Could you check a few things on this drawing? It's one solid part, dimensions in mm from its lowest x, y, z. A direction names the side the tool comes from. Coordinates: 2 decimals unless noted, no trailing zeros. Order: outer loops, then holes, each group sorted by start corner. A loop starts at its lowest first (then second) coordinate and runs counter-clockwise, first axis right, second up.
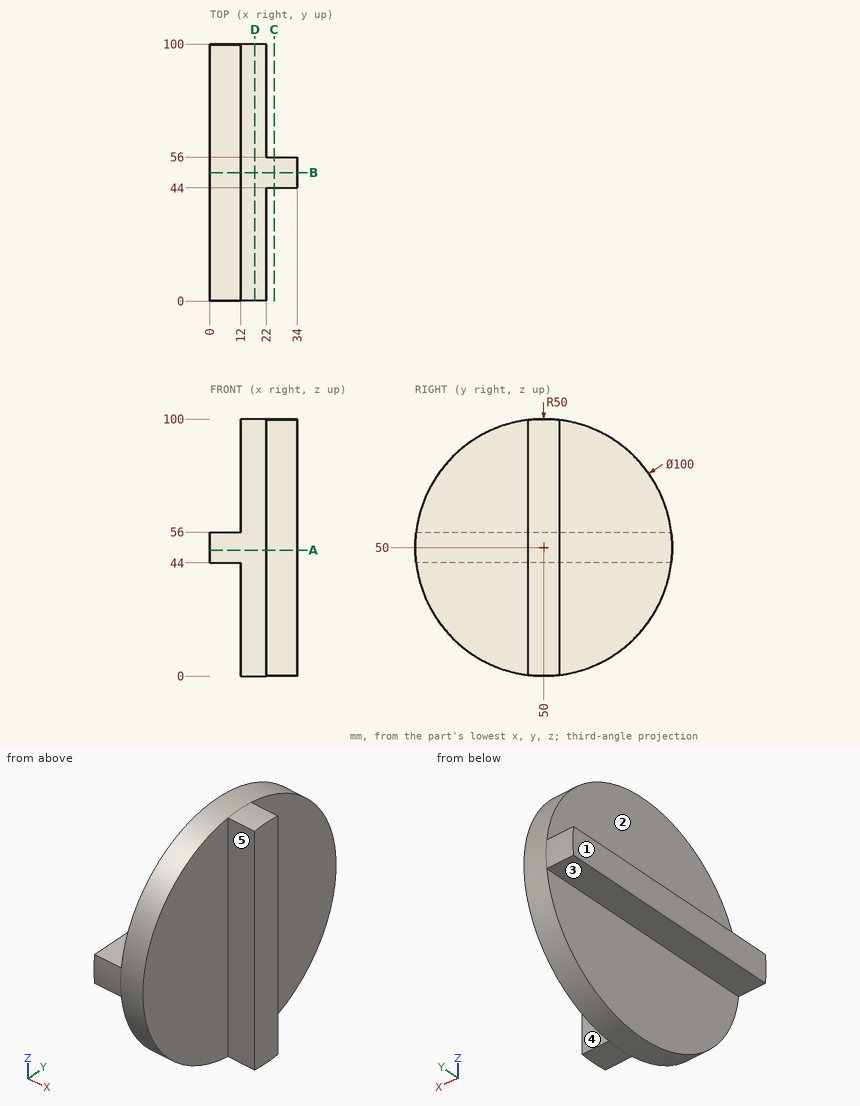
1. Imagine slicing it at C-C on x = 25. Please give me the cut outline in (y, z), then the cut area to 3 significant figures.
Completed:
outline: (44, 0.36) arc R50 ccw to (56, 0.36) - (56, 99.64) arc R50 ccw to (44, 99.64) - close
area: 1,200 mm2
2. On a 3-axis mill with a long thin cutter (end or side, diameter ignored), from which of +Z, -Z, +X, -X, +Y, -Y can I reach the whole of each face in a straight line? I mean the marked faces 1, 2, 3, 4 and 5. Say none if no direction works.
Completed:
face 1: +Z, -Z, -X, +Y, -Y
face 2: +Z, -X, +Y, -Y
face 3: -Z, -X, +Y, -Y
face 4: +Z, -Z, +X, +Y
face 5: +Z, -Z, +X, -Y
3. Imagine slicing it at A-A on z = 49. Please give me the cut outline in (x, y).
Completed:
outline: (0, 0.01) - (22, 0.01) - (22, 44) - (34, 44) - (34, 56) - (22, 56) - (22, 99.99) - (0, 99.99) - close
4. Please list where these lines run through material, in increasing order: probe 1 along X at (y, z) = (67.5, 70); probe 2 along X at (y, z) = (48, 30); probe 3 along Y at (x, z) = (30.5, 87.5).
Completed:
probe 1: x = 12 to 22
probe 2: x = 12 to 34
probe 3: y = 44 to 56
5. Imagine slicing it at B-B on y = 50. Please give me the cut outline in (x, z).
Completed:
outline: (0, 44) - (12, 44) - (12, 0) - (34, 0) - (34, 100) - (12, 100) - (12, 56) - (0, 56) - close
6. Imagine slicing it at D-D on x = 17.5. Please give me the cut outline in (y, z).
Completed:
outline: circle Ø100 at (50, 50)
7. I'm going to push flat-ended pins straight in: pin 1 (22 mm diameter, centred on y = 51, z = 77.5, fed in from -X); pin 2 (12 mm diameter, centred on x = 11.5, y = 86, fed in from +Z); pin 3 (13 mm diameter, centred on x = 30, z = 54, fed in from +Y). Where does each tip first touch, or does it pass through?
Completed:
pin 1: stops at x = 12
pin 2: stops at z = 89.98
pin 3: stops at y = 56
